Could you check a few things on this model? Use its own coordinates, in mm. A direction names the side the tool comes from. Give positions to 0.01 mm unless a question says otherwise; leave off trailing zeros. Loops run counter-clockwise (first coordinate to the right, second up) from the corner with the lowest first, then second, coordinate; pieces in that order, holes last. Notation, with made-up numbers: M -9,55.25 L 15,55.25 A23 ccw 15,84.25 Z; hole C -24.75,86.5 d10. An arc over 180 degrees is marked long. Answer in a Markdown table with one row per item. Add a question column.
```python
from build123d import *

# Parameters (mm, degrees)
SKETCH_W          = 9.5
SKETCH_H          = 11.1
PAD_DEPTH         = 2.5
POCKET_DEPTH      = 0.8
SKETCH002_R       = 0.8
PAD001_DEPTH      = 0.4
SKETCH003_R       = 0.8
PAD002_DEPTH      = 0.4
FILLET_R          = 0.2
SKETCH004_W       = 1.25
SKETCH004_H       = 0.7
POCKET001_DEPTH   = 9.5
FILLET001_R       = 1
FILLET002_R       = 0.5
PAD003_DEPTH      = 0.8
PAD003_DEPTH_BACK = 0.8


with BuildPart() as part:
    # Sketch → Pad (new body)
    with BuildSketch(Plane.XZ):
        with Locations((0, -0.7)):
            Rectangle(SKETCH_W, SKETCH_H)
    extrude(amount=PAD_DEPTH)

    # Sketch001 (on Face6 of Pad) → Pocket (cut)
    with BuildSketch(Plane.XZ.offset(2.5)):
        with BuildLine():
            Line((3.42, -2.28), (4.75, -2.28))
            Line((4.75, -2.28), (4.75, -6.25))
            Line((4.75, -6.25), (2.42, -6.25))
            Line((2.42, -6.25), (2.42, -3.28))
            ThreePointArc((3.42, -2.28), (2.712893, -2.572893), (2.42, -3.28))
        make_face()
        with BuildLine():
            Line((-4.75, 4.85), (-4.75, 2.28))
            Line((-4.75, 2.28), (-3.42, 2.28))
            ThreePointArc((-3.42, 2.28), (-2.712893, 2.572893), (-2.42, 3.28))
            Line((-2.42, 4.85), (-2.42, 3.28))
            Line((-4.75, 4.85), (-2.42, 4.85))
        make_face()
    extrude(amount=-POCKET_DEPTH, mode=Mode.SUBTRACT)

    # Sketch002 (on Face9 of Pocket) → Pad001 (join)
    with BuildSketch(Plane.XZ.offset(1.7)):
        with Locations((3.8, -3.65)):
            Circle(SKETCH002_R)
    extrude(amount=PAD001_DEPTH)

    # Sketch003 (on Face6 of Pad001) → Pad002 (join)
    with BuildSketch(Plane.XZ.offset(1.7)):
        with Locations((-3.8, 3.65)):
            Circle(SKETCH003_R)
    extrude(amount=PAD002_DEPTH)

    # Fillet
    fillet_edges = [part.edges().sort_by_distance(p)[0] for p in [
        (-4.6, -2.1, 3.65),
        (3, -2.1, -3.65),
    ]]
    fillet(fillet_edges, radius=FILLET_R)

    # Sketch004 (on Face13 of Fillet) → Pocket001 (cut)
    with BuildSketch(Plane(origin=(4.75, 0, 0), x_dir=(0, 0, 1), z_dir=(1, 0, 0))):
        with Locations((-5.625, 0.35)):
            Rectangle(SKETCH004_W, SKETCH004_H)
    extrude(amount=-POCKET001_DEPTH, mode=Mode.SUBTRACT)

    # Fillet001
    fillet001_edges = [part.edges().sort_by_distance(p)[0] for p in [
        (4.75, -1.25, 4.85),
        (-4.75, -0.85, 4.85),
    ]]
    fillet(fillet001_edges, radius=FILLET001_R)

    # Fillet002
    fillet002_edges = [part.edges().sort_by_distance(p)[0] for p in [
        (-4.75, -1.6, -6.25),
        (4.75, -1.2, -6.25),
    ]]
    fillet(fillet002_edges, radius=FILLET002_R)

    # Sketch005 (on Face5 of Fillet002) → Pad003 (join, two sides)
    with BuildSketch(Plane.XZ.offset(2.5)) as pad003_sk:
        with BuildLine():
            Line((-0.8, -5.6), (0.8, -5.6))
            ThreePointArc((1, -5.8), (0.941421, -5.658579), (0.8, -5.6))
            Line((1, -5.8), (1, -6.2))
            ThreePointArc((0.8, -6.4), (0.941421, -6.341421), (1, -6.2))
            Line((0.8, -6.4), (-0.8, -6.4))
            ThreePointArc((-1, -6.2), (-0.941421, -6.341421), (-0.8, -6.4))
            Line((-1, -6.2), (-1, -5.8))
            ThreePointArc((-0.8, -5.6), (-0.941421, -5.658579), (-1, -5.8))
        make_face()
    extrude(amount=PAD003_DEPTH)
    extrude(pad003_sk.sketch, amount=-PAD003_DEPTH_BACK)


solid = part.part
```
Item 1: For faces 1 (the face through (-2.8, -1.7, 3.6)), 2 (the face through (4, -2.1, -4)), 3 (the face through (-4, -2.1, 4)), 4 (the face through (0, -3, -6.4)), which set-ups out of +Z, -Z, +X, -X, +Y, -Y let a thin tool reach every point of the face, with its end or its side?
Item 2: If we mould it in two halves opening along Z, with no side actions, what happens to faces 5 (the face through (4, -1.7, -5)), 6 (the face through (-4.465, -0.862, 4.549)), 7 (the face through (0, -0.7, -6)), 8 (the face through (-2.721, -2.106, 2.565))? For each: +Z half, -Z half, draft (parallel to the pull), parting line (faces both ways), or undercut.
Item 3: Suppose I cut it at C-C (x = 0.5). List the corners of the cut face in (y, z) for me.
Item 4: Suppose I cut it at D-D (y = -0.55). List the corners of the cut face in (x, z) for me, then the cut area to 3 significant figures.
Item 5: For P1, Ø0.6, axis at x = 4, z = -4, coming from the -Y side; P2, Ø1.5, axis at x = -2.5, y = -3, coming from the -Z side; P3, Ø2.5, axis at x = -3, z = 3, coming from the -Y side, each with a flat end and sliding along its axis, tell me the tip position at first contact or that it passes through.
Item 6: Suppose I cut it at A-A (y = -2.8). List the corners of the cut face in (x, z) for me, then the cut area to 3 significant figures.
Item 7: I need wall thicknesses on L1, parallel to Y at x = -3.25, z = -0.25; L2, parallel to Z at x = -1, y = -0.95; L3, parallel to Y at x = -4.5, z = 4.25. Which ranges of each line are inside material? Lowest first, please.
Item 8: Suppose I cut it at B-B (z = -3.65). List the corners of the cut face in (x, y) for me.
Values found:
| question | item | result |
|---|---|---|
| 1 | face 1 | -Y |
| 1 | face 2 | -Z, +X, -Y |
| 1 | face 3 | +Z, -X, -Y |
| 1 | face 4 | -Z, +X, -X, +Y, -Y |
| 2 | face 5 | undercut |
| 2 | face 6 | +Z half |
| 2 | face 7 | draft |
| 2 | face 8 | undercut |
| 3 | outline | M -3.3,-6.4 L -1.7,-6.4 L -1.7,-6.25 L -0.7,-6.25 L -0.7,-5 L 0,-5 L 0,4.85 L -2.5,4.85 L -2.5,-5.6 L -3.3,-5.6 Z |
| 4 | outline | M -4.75,-5 L 4.75,-5 L 4.75,3.85 A1 ccw 3.75,4.85 L -3.75,4.85 A1 ccw -4.75,3.85 Z |
| 4 | area | 93.1 mm² |
| 5 | P1 | y = -2.1 |
| 5 | P2 | z = -6.25 |
| 5 | P3 | y = -2.5 |
| 6 | outline | M -1,-6.2 A0.2 ccw -0.8,-6.4 L 0.8,-6.4 A0.2 ccw 1,-6.2 L 1,-5.8 A0.2 ccw 0.8,-5.6 L -0.8,-5.6 A0.2 ccw -1,-5.8 Z |
| 6 | area | 1.57 mm² |
| 7 | L1 | -2.5 to 0 |
| 7 | L2 | -6.25 to 4.85 |
| 7 | L3 | -1.7 to 0 |
| 8 | outline | M -4.75,-2.5 L 2.42,-2.5 L 2.42,-1.7 L 3,-1.7 L 3,-1.9 A0.2 ccw 3.2,-2.1 L 4.4,-2.1 A0.2 ccw 4.6,-1.9 L 4.6,-1.7 L 4.75,-1.7 L 4.75,0 L -4.75,0 Z |
